from build123d import *

# Parameters (mm, degrees)
SKETCH_1_W             = 130
SKETCH_1_H             = 38
EXTRUDE_1_DEPTH        = 1.5
SKETCH_2_W             = 3.5
SKETCH_2_H             = 10
EXTRUDE_2_DEPTH        = 3
CUT_EXTRUDE_2_DEPTH    = 4
SKETCH_3_R             = 0.75
CUT_EXTRUDE_1_DEPTH    = 4
FILLET_1_R             = 0.5
CUT_EXTRUDE_3_DEPTH    = 4
FILLET_2_R             = 1
CUT_EXTRUDE_4_DEPTH    = 4
CUT_EXTRUDE_6_DEPTH    = 4
SKETCH_9_R             = 0.6
CUT_EXTRUDE_7_DEPTH    = 4
FILLET_3_R             = 0.5
CUT_EXTRUDE_8_DEPTH    = 4
FILLET_4_R             = 1
CHAMFER_1_SIZE         = 3
CHAMFER_1_EDGE_2_SIZE2 = 3.330793123
CHAMFER_1_EDGE_2_SIZE  = 3


with BuildPart() as part:
    # 草图1 → 凸台-拉伸1 (new body, symmetric)
    with BuildSketch(Plane.XY):
        Rectangle(SKETCH_1_W, SKETCH_1_H)
    extrude(amount=EXTRUDE_1_DEPTH, both=True)

    # 草图2 → 凸台-拉伸2 (add)
    with BuildSketch(Plane.XY.offset(1.5)):
        with Locations((66.75, 10)):
            Rectangle(SKETCH_2_W, SKETCH_2_H)
        with Locations((66.75, -10)):
            Rectangle(SKETCH_2_W, SKETCH_2_H)
    extrude(amount=-EXTRUDE_2_DEPTH)

    # 草图4 → 切除-拉伸2 (cut, through all)
    with BuildSketch(Plane.XY.offset(1.5)):
        Polygon((48.85, 12.5), (54.95, 12.5), (54.95, 7.5), (51.95, 7.5), (51.95, -7.5), (54.95, -7.5), (54.95, -12.5), (48.85, -12.5), align=None)
    extrude(amount=-CUT_EXTRUDE_2_DEPTH, mode=Mode.SUBTRACT)

    # 草图3 → 切除-拉伸1 (cut, through all)
    with BuildSketch(Plane.XY.offset(1.5)):
        with Locations((65, 15.75)):
            Circle(SKETCH_3_R)
        with Locations((65, 4.25)):
            Circle(SKETCH_3_R)
        with Locations((65, -4.25)):
            Circle(SKETCH_3_R)
        with Locations((65, -15.75)):
            Circle(SKETCH_3_R)
        with Locations((54.95, 8.25)):
            Circle(SKETCH_3_R)
        with Locations((54.2, 12.5)):
            Circle(SKETCH_3_R)
        with Locations((48.85, 11.75)):
            Circle(SKETCH_3_R)
        with Locations((48.85, -11.75)):
            Circle(SKETCH_3_R)
        with Locations((54.95, -8.25)):
            Circle(SKETCH_3_R)
        with Locations((54.2, -12.5)):
            Circle(SKETCH_3_R)
    extrude(amount=-CUT_EXTRUDE_1_DEPTH, mode=Mode.SUBTRACT)

    # 圆角1
    fillet_1_edges = [part.edges().sort_by_distance(p)[0] for p in [
        (68.5, 15, 0),
        (68.5, 5, 0),
        (68.5, -5, 0),
        (68.5, -15, 0),
        (51.95, 7.5, 0),
        (51.95, -7.5, 0),
    ]]
    fillet(fillet_1_edges, radius=FILLET_1_R)

    # 草图5 → 切除-拉伸3 (cut, through all)
    with BuildSketch(Plane.XY.offset(1.5)):
        Polygon((-65, -19), (-65, -14), (35.804501844, -14), (40, -19), align=None)
    extrude(amount=-CUT_EXTRUDE_3_DEPTH, mode=Mode.SUBTRACT)

    # 圆角2
    fillet_2_edges = [part.edges().sort_by_distance(p)[0] for p in [
        (40, -19, 0),
        (35.804501844, -14, 0),
    ]]
    fillet(fillet_2_edges, radius=FILLET_2_R)

    # 草图6 → 切除-拉伸4 (cut, through all)
    with BuildSketch(Plane.XY.offset(1.5)):
        Polygon((-65, 9), (40, 19), (-65, 19), align=None)
    extrude(amount=-CUT_EXTRUDE_4_DEPTH, mode=Mode.SUBTRACT)

    # 草图8 → 切除-拉伸6 (cut, through all)
    with BuildSketch(Plane(origin=(0, 0, -1.5), x_dir=(-1, 0, 0), z_dir=(0, 0, -1))):
        Polygon((29.975, -6), (29.975, -9), (23.875, -9), (23.875, 4), (29.975, 4), (29.975, 1), (26.975, 1), (26.975, -6), align=None)
        Polygon((58.025, 1), (58.025, -6), (55.025, -6), (55.025, -9), (61.125, -9), (61.125, 4), (55.025, 4), (55.025, 1), align=None)
    extrude(amount=-CUT_EXTRUDE_6_DEPTH, mode=Mode.SUBTRACT)

    # 草图9 → 切除-拉伸7 (cut, through all)
    with BuildSketch(Plane(origin=(0, 0, -1.5), x_dir=(-1, 0, 0), z_dir=(0, 0, -1))):
        with Locations((29.975, 1.6)):
            Circle(SKETCH_9_R)
        with Locations((29.975, -6.6)):
            Circle(SKETCH_9_R)
        with Locations((29.375, -9)):
            Circle(SKETCH_9_R)
        with Locations((29.375, 4)):
            Circle(SKETCH_9_R)
        with Locations((23.875, 3.4)):
            Circle(SKETCH_9_R)
        with Locations((23.875, -8.4)):
            Circle(SKETCH_9_R)
        with Locations((55.025, -6.6)):
            Circle(SKETCH_9_R)
        with Locations((55.625, -9)):
            Circle(SKETCH_9_R)
        with Locations((55.025, 1.6)):
            Circle(SKETCH_9_R)
        with Locations((55.625, 4)):
            Circle(SKETCH_9_R)
        with Locations((61.125, 3.4)):
            Circle(SKETCH_9_R)
        with Locations((61.125, -8.4)):
            Circle(SKETCH_9_R)
    extrude(amount=-CUT_EXTRUDE_7_DEPTH, mode=Mode.SUBTRACT)

    # 圆角3
    fillet_3_edges = [part.edges().sort_by_distance(p)[0] for p in [
        (-26.975, -6, 0),
        (-26.975, 1, 0),
        (-58.025, 1, 0),
        (-58.025, -6, 0),
    ]]
    fillet(fillet_3_edges, radius=FILLET_3_R)

    # 草图11 → 切除-拉伸8 (cut, through all)
    with BuildSketch(Plane(origin=(0, 0, -1.5), x_dir=(-1, 0, 0), z_dir=(0, 0, -1))):
        with BuildLine():
            Line((21.392298894, -14), (18.875, -11))
            Line((18.875, -11), (-33.287202951, -11))
            Line((-33.287202951, -11), (-36.104238629, -14.35721239))
            ThreePointArc((-36.104238629, -14.35721239), (-35.760812448, -14.093692213), (-35.338194186, -14))
            Line((-35.338194186, -14), (21.392298894, -14))
        make_face()
    extrude(amount=-CUT_EXTRUDE_8_DEPTH, mode=Mode.SUBTRACT)

    # 圆角4
    fillet_4_edges = [part.edges().sort_by_distance(p)[0] for p in [
        (-21.392298894, -14, 0),
        (33.287202951, -11, 0),
        (-18.875, -11, 0),
    ]]
    fillet(fillet_4_edges, radius=FILLET_4_R)

    # 倒角1
    chamfer_1_edges = [part.edges().sort_by_distance(p)[0] for p in [
        (-65, -14, 0),
    ]]
    chamfer(chamfer_1_edges, length=CHAMFER_1_SIZE)

    # 倒角1 edge 2
    chamfer_1_edge_2_edges = [part.edges().sort_by_distance(p)[0] for p in [
        (-65, 9, 0),
    ]]
    chamfer(chamfer_1_edge_2_edges, length=CHAMFER_1_EDGE_2_SIZE, length2=CHAMFER_1_EDGE_2_SIZE2)


solid = part.part
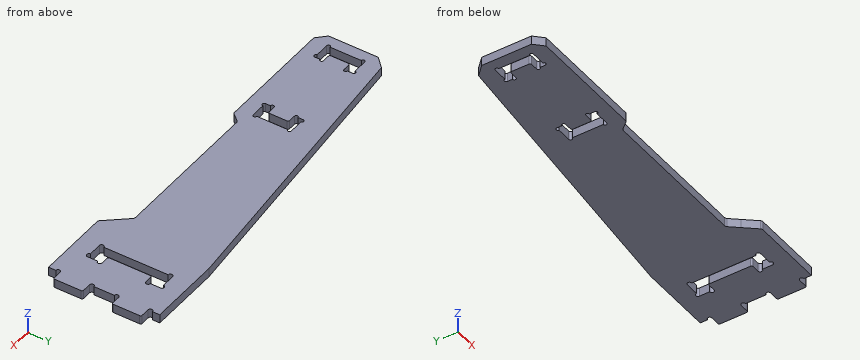
For this review, take the finished solid that the model builds, in its own axes (mm). Give positions to 0.01 mm unless a question says otherwise; leave off trailing zeros. Write each loop counter-clockwise with the first axis right and the second up, starting at its lowest first coordinate (ties: lowest second). Pieces come first, ordered by that corner, then holes. Notation, with made-up numbers: (-36.75, 73) -> (2.25, 73) arc R6 ccw to (2.25, 77) -> close; hole circle Ø9 at (-12.75, 62). An arc over 180 degrees is marked (long way). Use CSV: the item, a comma, the result in double quotes.
Q1. Take a section at A-A, the plane z = -1. State how many separate pieces and enclosed holes the cut face has, then the cut area to 3 significant figures.
Conclusion:
separate pieces,"1"
enclosed holes,"3"
area,"3,560 mm2"
Q2. To check wall thickness, follow probe 1 along X at (y, z) = (-2.5, -0.25) (3 decimals); probe 2 along X at (y, z) = (-7, -1.15) (3 decimals); probe 3 along Y at (x, z) = (-56, -0.1). State the ranges of each line that lie inside material, in increasing order. Write a range as [from, to].
Conclusion:
probe 1,"[-65, -61.125], [-58.025, -26.975], [-23.875, 48.85], [51.95, 65]"
probe 2,"[-65, -61.125], [-54.578, -30.422], [-23.875, 48.85], [51.95, 68.5]"
probe 3,"[-14, -9.47], [-6, 1], [4.47, 9.86]"
Q3. For P1, Ø0.9, axis at x = -57.5, z = 0.5, coming from the +Y side; P2, Ø0.9, axis at x = -58, z = 0, coming from the -Y side; P3, Ø0.8, axis at y = 18, z = -0.5, coming from the +X side, all flat-tipped, find the tip position at first contact; note any pin that passes through.
Conclusion:
P1,"y = 9.76"
P2,"y = -14"
P3,"x = 65"
Q4. Take a section at C-C, the plane x = -15. Write out the cut boundary in (y, z).
Conclusion:
outline,"(-11, -1.5) -> (13.76, -1.5) -> (13.76, 1.5) -> (-11, 1.5) -> close"
Q5. Take a section at B-B, the plane x = -35. Write out the cut boundary in (y, z).
Conclusion:
outline,"(-14, -1.5) -> (11.86, -1.5) -> (11.86, 1.5) -> (-14, 1.5) -> close"
